from build123d import *

# Parameters (mm, degrees)
SKICA1_R                 = 2
P_IDAT_VYSUNUT_M1_DEPTH  = 1
SKICA2_R                 = 1.15
ODEBRAT_VYSUNUT_M1_DEPTH = 2
SKICA3_R                 = 3
SKICA3_R_2               = 2
P_IDAT_VYSUNUT_M2_DEPTH  = 3
KRUHOV_POLE1_COUNT       = 4


with BuildPart() as part:
    # Skica1 → Přidat vysunutím1 (new body)
    with BuildSketch(Plane(origin=(0, 0, 0), x_dir=(1, 0, 0), z_dir=(0, 1, 0))):
        with BuildLine():
            Line((-12.62, 1.495192295), (-2.5, 2.307395517))
            Line((-2.5, 2.307395517), (-1.687796778, 12.427395517))
            ThreePointArc((-1.687796778, 12.427395517), (-0.192604483, 13.807395517), (1.302587813, 12.427395517))
            Line((1.302587813, 12.427395517), (2.114791035, 2.307395517))
            Line((2.114791035, 2.307395517), (12.234791035, 1.495192295))
            ThreePointArc((12.234791035, 1.495192295), (13.614791035, 0), (12.234791035, -1.495192295))
            Line((12.234791035, -1.495192295), (2.114791035, -2.307395517))
            Line((2.114791035, -2.307395517), (1.302587813, -12.427395517))
            ThreePointArc((1.302587813, -12.427395517), (-0.192604483, -13.807395517), (-1.687796778, -12.427395517))
            Line((-1.687796778, -12.427395517), (-2.5, -2.307395517))
            Line((-2.5, -2.307395517), (-12.62, -1.495192295))
            ThreePointArc((-12.62, -1.495192295), (-14, 0), (-12.62, 1.495192295))
        make_face()
        Circle(SKICA1_R, mode=Mode.SUBTRACT)
    extrude(amount=P_IDAT_VYSUNUT_M1_DEPTH)

    # Skica2 → Odebrat vysunutím1 (cut)
    with BuildSketch(Plane(origin=(0, 1, 0), x_dir=(1, 0, 0), z_dir=(0, 1, 0))):
        with Locations((-8.5, 0)):
            Circle(SKICA2_R)
        with Locations((8.5, 0)):
            Circle(SKICA2_R)
    odebrat_vysunut_m1 = extrude(amount=-ODEBRAT_VYSUNUT_M1_DEPTH, mode=Mode.SUBTRACT)

    # Skica3 → Přidat vysunutím2 (add)
    with BuildSketch(Plane(origin=(0, 1, 0), x_dir=(1, 0, 0), z_dir=(0, 1, 0))):
        Circle(SKICA3_R)
        Circle(SKICA3_R_2, mode=Mode.SUBTRACT)
    extrude(amount=P_IDAT_VYSUNUT_M2_DEPTH)

    # Kruhové pole1: Odebrat vysunutím1 ×4 about axis
    kruhov_pole1_axis = Axis((0, 0, 0), (0, 1, 0))
    for i in range(1, KRUHOV_POLE1_COUNT):
        add(odebrat_vysunut_m1.rotate(kruhov_pole1_axis, i * 360 / KRUHOV_POLE1_COUNT), mode=Mode.SUBTRACT)


solid = part.part
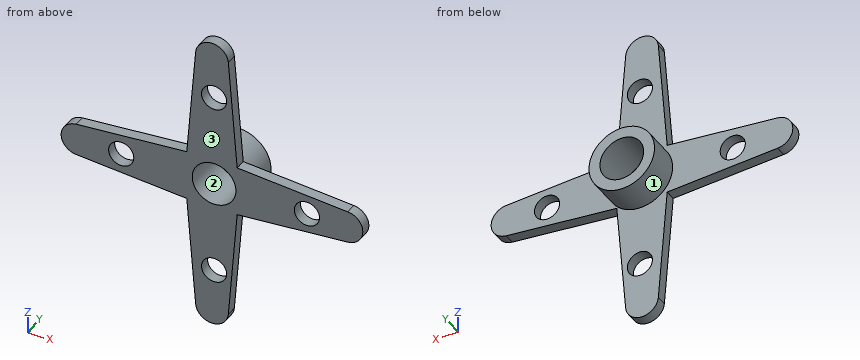
The model under review builds one solid part; all positions refer to its coordinate system, in mm. Face numbers are marked on the shaded views. Round coordinates to 2 decimals unless told otherwise and drop trailing zeros. Order: outer loops, then holes, each group sorted by start corner. A loop starts at its lowest first (then second) coordinate and runs counter-clockwise, first axis right, second up. Notation, with made-up numbers: (37, -4.5) -> (76, -4.5) arc R19 ccw to (76, 22.5) -> close; hole circle Ø5 at (80.25, 38.25). An arc over 180 degrees is marked (long way). Write item = value, one per line. Start each with the question number.
Item 1: Mouldability with a two-part tool opening along X and no side actions: class the marked faces 1, 2 and 3 as released by +X, released by -X, zero draft, split by the parting line, or undercut.
Item 2: Clearance check with flat-ended pins moving along their axes: pin 1 Ø12 at (x, z) = (-8.5, -5.5) entering from +Y; pin 2 Ø2 at (x, z) = (0, 8.5) entering from -Y; pin 3 Ø3 at (x, z) = (0, -8.5) entering from -Y; pin 4 Ø2 at (y, z) = (0.5, -4.5) entering from +X. State where each tip first meets the part, or that it passes through.
Item 3: Consider section C-C on z = -8.5. Write out the cut boundary in (x, y), plus the area to 3 significant figures.
Item 4: Consider section B-B on x = 8.5. Write out the cut boundary in (y, z), plus the area to 3 significant figures.
Item 5: For line 1 along Z through (x, y) = (0, 2.7); line 2 along X through (y, z) = (0.4, 7.75), list the stretches that pass through material, from the lowest coordinate up.
Item 6: Consider section A-A on z = 0. Write out the cut boundary in (x, y).
Item 7: Consider section D-D on x = 0. Write out the cut boundary in (y, z).
Conclusion:
q1.face_1 = split by the parting line
q1.face_2 = undercut
q1.face_3 = zero draft
q2.pin_1 = 1
q2.pin_2 = through
q2.pin_3 = 0
q2.pin_4 = 2.02
q3.outline = (-2, 0) -> (-1.15, 0) -> (-1.15, 1) -> (-2, 1) -> close; (1.15, 0) -> (1.62, 0) -> (1.62, 1) -> (1.15, 1) -> close
q3.area = 1.32 mm2
q4.outline = (0, -1.79) -> (1, -1.79) -> (1, -1.15) -> (0, -1.15) -> close; (0, 1.15) -> (1, 1.15) -> (1, 1.79) -> (0, 1.79) -> close
q4.area = 1.29 mm2
q5.line_1 = -3 to -2, 2 to 3
q5.line_2 = -2.06 to -0.87, 0.87 to 1.68
q6.outline = (-14, 0) -> (-9.65, 0) -> (-9.65, 1) -> (-14, 1) -> close; (-7.35, 0) -> (-2, 0) -> (-2, 4) -> (-3, 4) -> (-3, 1) -> (-7.35, 1) -> close; (2, 0) -> (7.35, 0) -> (7.35, 1) -> (3, 1) -> (3, 4) -> (2, 4) -> close; (9.65, 0) -> (13.61, 0) -> (13.61, 1) -> (9.65, 1) -> close
q7.outline = (0, -13.79) -> (1, -13.79) -> (1, -9.65) -> (0, -9.65) -> close; (0, -7.35) -> (1, -7.35) -> (1, -3) -> (4, -3) -> (4, -2) -> (0, -2) -> close; (0, 2) -> (4, 2) -> (4, 3) -> (1, 3) -> (1, 7.35) -> (0, 7.35) -> close; (0, 9.65) -> (1, 9.65) -> (1, 13.79) -> (0, 13.79) -> close
